For this review, use the dimensioned drawing (mm, ordinates from the lowest corner) and the shaded views. A direction names the side the tool comes from. Give positions to 0.01 mm unless a question says otherwise; leave off trailing zeros. Loops run counter-clockwise (first coordinate to the right, second up) from the corner with the lowest first, then second, coordinate; pieces in that order, holes last. Notation, with made-up numbers: (-4.75, 10.5) -> (23.25, 10.5) arc R28 cw to (23.25, 28.5) -> close; hole circle Ø5 at (-33, -27.5). An arc over 180 degrees is marked (long way). Use a Markdown table: item, result. Add a question column.
1. Add section C-C (y = 2). State the section outline as (x, z) points.
2. Add section D-D (x = 15.5). State the section outline as (y, z) points, and give its area (3 significant figures).
3. Add section B-B (x = 4). State the section outline as (y, z) points, and give its area (3 significant figures).
4. For pin 1 Ø1.5 at (x, z) = (14, 5) entering from +Y, flat-tipped, find the tip position at first contact; note if it passes through.
5. For the marked faces 5, 6 and 7, list the 3-axis set-ups (+Z, -Z, +X, -X, +Y, -Y) from which the entire face can be reached by the end or side of a thin tool; tool diameter is ignored.
6. Draft analysis for pull direction X (two halves, no side actions). For the marked faces 1, 2, 3 and 4, state which applies: pulls with the +X half, pulls with the -X half, needs draft (parallel to the pull), parting line crosses it, or undercut.
7. To check wall thickness, follow line 1 (Z direction, x = 7.75, y = 9.5); line 2 (X direction, y = 8.5, z = 8.5); line 3 (X direction, y = 1.5, z = 7.5). State the ranges of each line that lie inside material, in increasing order.
8. Add section A-A (z = 7.75). State the section outline as (x, y) points.
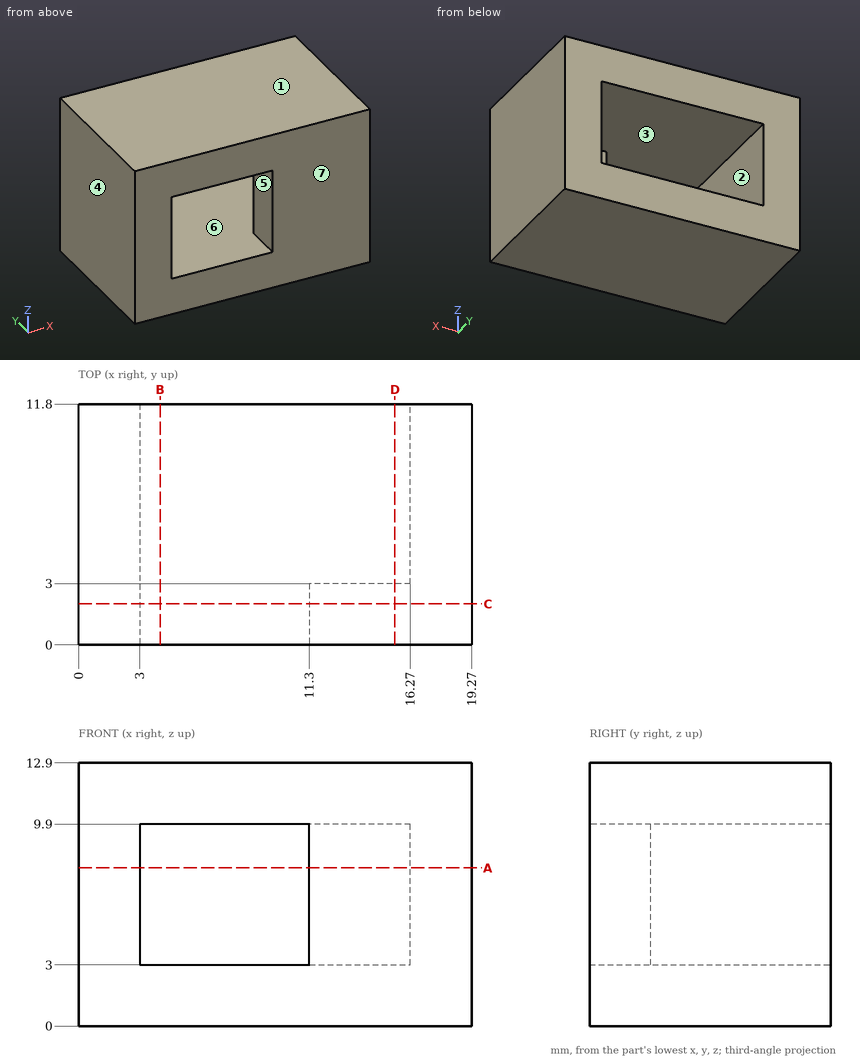
Taken from the geometry:
| question | item | result |
|---|---|---|
| 1 | outline | (0, 0) -> (19.27, 0) -> (19.27, 12.9) -> (0, 12.9) -> close; hole (3, 3) -> (11.3, 3) -> (11.3, 9.9) -> (3, 9.9) -> close |
| 2 | outline | (0, 0) -> (11.8, 0) -> (11.8, 3) -> (3, 3) -> (3, 9.9) -> (11.8, 9.9) -> (11.8, 12.9) -> (0, 12.9) -> close |
| 2 | area | 91.5 mm^2 |
| 3 | outline | (0, 0) -> (11.8, 0) -> (11.8, 3) -> (0, 3) -> close; (0, 9.9) -> (11.8, 9.9) -> (11.8, 12.9) -> (0, 12.9) -> close |
| 3 | area | 70.8 mm^2 |
| 4 | pin 1 | stops at y = 3 |
| 5 | face 5 | +Y, -Y |
| 5 | face 6 | +Y |
| 5 | face 7 | +Z, -Z, +X, -X, -Y |
| 6 | face 1 | needs draft |
| 6 | face 2 | undercut |
| 6 | face 3 | undercut |
| 6 | face 4 | pulls with the -X half |
| 7 | line 1 | z = 0 to 3, 9.9 to 12.9 |
| 7 | line 2 | x = 0 to 3, 16.27 to 19.27 |
| 7 | line 3 | x = 0 to 3, 11.3 to 19.27 |
| 8 | outline | (0, 0) -> (3, 0) -> (3, 11.8) -> (0, 11.8) -> close; (11.3, 0) -> (19.27, 0) -> (19.27, 11.8) -> (16.27, 11.8) -> (16.27, 3) -> (11.3, 3) -> close |
